Work out the finished part from the listing and answer in its coordinate system (mm). A direction names the side the tool comes from. Coordinates: 2 decimals unless noted, no trailing zeros. Order: outer loops, then holes, each group sorted by start corner. A loop starts at its lowest first (then second) coordinate and runs counter-clockwise, first axis right, second up.
1. Flat-ended cylindrical pins translate along their axes: pin 1 Ø12 at (y, z) = (-11, 48) entering from -X; pin 2 Ø5 at (x, z) = (24.5, 45.5) entering from +Y; pin 3 Ø12 at (x, z) = (31.5, 21) entering from -Y; pin 4 Ø15 at (x, z) = (32, 38.5) entering from +Y. Find the tip coordinate at first contact, or state that the pin passes through.
2. The part is cut by section C-C, the plane y = -23. Give the vertices of the cut face in (x, z).
3. Find the intervals of material crossed by probe 1 along Z at (x, y) = (35, -31); probe 2 along Y at (x, z) = (18.5, 23), in increasing order.
4. The part is cut by section D-D, the plane z = 48. Give the vertices of the cut face in (x, y), then the cut area to 3 significant figures.
5. The part is cut by section A-A, the plane y = -44. Give the vertices of the cut face in (x, z).
6. A tool of negligible diameter and unlimited length cuts with its end or side. For faces 5 (the cylindrical face through (49.793, -4.54, 23.298)), 6 (the flat face through (19, -23, 3)), 7 (the cylindrical face through (46.7, 4.93, 18.45)), from which of +Z, -Z, +X, -X, +Y, -Y can it reach the whole face along a straight path? Write none if from no direction.
7. The part is cut by section B-B, the plane x = 6. Give the vertices of the cut face in (y, z), then the cut area to 3 significant figures.
8. Determine the mould class of faces 1 (the cylindrical face through (5.479, -40.034, 53.521)), 2 (the flat face through (34, 25, 28)), 3 (the flat face through (24, -6, 27)), 4 (the flat face through (19, -23, 52)) for opening direction Y: +Y half, -Y half, draft (parallel to the pull), parting line (faces both ways), or undercut.
```python
from build123d import *

# Parameters (mm, degrees)
F1_DEPTH = 55
F2_W     = 44
F2_H     = 49
F3_DEPTH = 50.001
F4_R     = 4
F5_DEPTH = 55
F6_R     = 16
F7_DEPTH = 25
F8_R     = 15


with BuildPart() as f1:
    # F0 (on Top) → F1 (new body)
    with BuildSketch(Plane.XY):
        with BuildLine():
            Line((0, 0), (0, -50))
            ThreePointArc((0, -50), (35.355339, -35.355339), (50, 0))
            Line((50, 0), (0, 0))
        make_face()
    extrude(amount=F1_DEPTH)

    # F2 (on face) → F3 (cut, through all)
    with BuildSketch(Plane(origin=(0, 0, 0), x_dir=(0, -1, 0), z_dir=(-1, 0, 0))):
        with Locations((28, 27.5)):
            Rectangle(F2_W, F2_H)
    extrude(amount=-F3_DEPTH, mode=Mode.SUBTRACT)

    # F4 (on face) → F5 (cut)
    with BuildSketch(Plane.XY.offset(55)):
        with Locations((6, -44)):
            Circle(F4_R)
    extrude(amount=-F5_DEPTH, mode=Mode.SUBTRACT)

    # F6 (on face) → F7 (join)
    with BuildSketch(Plane(origin=(0, 0, 0), x_dir=(-1, 0, 0), z_dir=(0, 1, 0))):
        with Locations((-34, 28.184593)):
            Circle(F6_R)
    extrude(amount=F7_DEPTH)

    # F8
    f8_edges = [f1.edges().sort_by_distance(p)[0] for p in [
        (50, 25, 28.184593),
    ]]
    fillet(f8_edges, radius=F8_R)


solid = f1.part
```
Geometry says:
1. pin 1: stops at x = 0
1. pin 2: stops at y = 0
1. pin 3: stops at y = -6
1. pin 4: stops at y = 24.87
2. outline: (0, 0) - (44.4, 0) - (44.4, 3) - (0, 3) - close; (0, 52) - (44.4, 52) - (44.4, 55) - (0, 55) - close
3. probe 1: z = 0 to 3, 52 to 55
3. probe 2: y = -6 to 0
4. outline: (0, -6) - (49.64, -6) arc R50 ccw to (50, 0) - (0, 0) - close
4. area: 299 mm2
5. outline: (0, 0) - (2, 0) - (2, 3) - (0, 3) - close; (0, 52) - (2, 52) - (2, 55) - (0, 55) - close; (10, 0) - (23.75, 0) - (23.75, 3) - (10, 3) - close; (10, 52) - (23.75, 52) - (23.75, 55) - (10, 55) - close
6. face 5: +Z, -Z, +X, -Y
6. face 6: +X, -X, -Y
6. face 7: +Y
7. outline: (-49.64, 0) - (-48, 0) - (-48, 3) - (-49.64, 3) - close; (-49.64, 52) - (-48, 52) - (-48, 55) - (-49.64, 55) - close; (-40, 0) - (0, 0) - (0, 55) - (-40, 55) - (-40, 52) - (-6, 52) - (-6, 3) - (-40, 3) - close
7. area: 544 mm2
8. face 1: undercut
8. face 2: +Y half
8. face 3: -Y half
8. face 4: draft
